Input: part model. Units: mm. Frame: model coordinates. A direction names the side the tool comes from. Give positions to 0.01 mm unless a question says otherwise; leave off trailing zeros. Order: outer loops, then holes, each group sorted by start corner. A loop starts at its lowest first (then second) coordinate and runs counter-clockwise, first axis right, second up. Notation, with made-up numbers: (82, 76) - (136, 76) arc R9 cw to (136, 86) - close; hole circle Ø10 at (7, 41.25). An arc over 180 degrees is marked (long way). Use a Markdown table: item, result.
from build123d import *

# Parameters (mm, degrees)
SKETCH013_W             = 28.2
SKETCH013_H             = 23.6
PAD004_DEPTH            = 2
SKETCH014_W             = 1.9812
SKETCH014_H             = 1.27
POCKET005_DEPTH         = 2
SKETCH015_R             = 4
SKETCH015_R_2           = 2.5
PAD005_DEPTH            = 8.6
SKETCH016_R             = 1.7
POCKET006_DEPTH         = 2
BODY002_PLACEMENT_ANGLE = 180


with BuildPart() as part:
    # Sketch013 → Pad004 (new body)
    with BuildSketch(Plane.XY):
        with Locations((0, -33.4375)):
            Rectangle(SKETCH013_W, SKETCH013_H)
    extrude(amount=PAD004_DEPTH)

    # Sketch014 (on Face6 of Pad004) → Pocket005 (cut)
    with BuildSketch(Plane.XY.offset(2)):
        with Locations((-6.1781, -26.6025)):
            Rectangle(SKETCH014_W, SKETCH014_H)
        with Locations((6.1781, -26.6025)):
            Rectangle(SKETCH014_W, SKETCH014_H)
    extrude(amount=-POCKET005_DEPTH, mode=Mode.SUBTRACT)

    # Sketch015 (on Face5 of Pocket005) → Pad005 (join)
    with BuildSketch(Plane.XY.offset(2)):
        with Locations((-6.1781, -26.6025)):
            Circle(SKETCH015_R)
        with Locations((-6.1781, -26.6025)):
            Circle(SKETCH015_R_2, mode=Mode.SUBTRACT)
        with Locations((6.1781, -26.6025)):
            Circle(SKETCH015_R)
        with Locations((6.1781, -26.6025)):
            Circle(SKETCH015_R_2, mode=Mode.SUBTRACT)
    extrude(amount=PAD005_DEPTH)

    # Sketch016 (on Face5 of Pad005) → Pocket006 (cut)
    with BuildSketch(Plane.XY.offset(2)):
        with Locations((-11, -42.2375)):
            Circle(SKETCH016_R)
        with Locations((11, -42.2375)):
            Circle(SKETCH016_R)
        with Locations((-11, -33.2375)):
            Circle(SKETCH016_R)
        with Locations((11, -33.2375)):
            Circle(SKETCH016_R)
    extrude(amount=-POCKET006_DEPTH, mode=Mode.SUBTRACT)


with BuildPart() as part_1:
    # Body002 placement: moved
    add(part.part.rotate(Axis((0, 0, 0), (0, 1, 0)), BODY002_PLACEMENT_ANGLE))


solid = part_1.part
1. Section query C-C (x = -3). Return loops of the section in (y, z).
Response:
| item | result |
|---|---|
| outline | (-45.24, -2) - (-29.03, -2) - (-29.03, -10.6) - (-24.17, -10.6) - (-24.17, -2) - (-21.64, -2) - (-21.64, 0) - (-45.24, 0) - close |
2. Section query B-B (z = -6.5). Return loops of the section in (x, y).
Response:
| item | result |
|---|---|
| outline | circle Ø8 at (-6.18, -26.6); circle Ø8 at (6.18, -26.6); hole circle Ø5 at (-6.18, -26.6); hole circle Ø5 at (6.18, -26.6) |
3. Section query A-A (x = 11). Return loops of the section in (y, z).
Response:
| item | result |
|---|---|
| outline | (-45.24, -2) - (-43.94, -2) - (-43.94, 0) - (-45.24, 0) - close; (-40.54, -2) - (-34.94, -2) - (-34.94, 0) - (-40.54, 0) - close; (-31.54, -2) - (-21.64, -2) - (-21.64, 0) - (-31.54, 0) - close |
4. Mould query, pull axis Y, two halves, no side actions, for faces 4 (the face through (-5.636, -29.043, -6.24)), 5 (the face through (-5.657, -22.637, -6.24)), 6 (the face through (-5.188, -27, -1)), 7 (the face through (-9, -27, -10.6)). Classes: pulls with the +Y half, pulls with the -Y half, needs draft (parallel to the pull), parting line crosses it, or undercut.
Response:
| item | result |
|---|---|
| face 4 | undercut |
| face 5 | parting line crosses it |
| face 6 | undercut |
| face 7 | needs draft |
5. Material intervals for line 1 along Y through (x, z) = (-11, -1.25); line 2 along Y through (x, z) = (-5.5, -1.5); line 3 along X through (y, z) = (-27.5, -7), sorted ascending.
Response:
| item | result |
|---|---|
| line 1 | y = -45.24 to -43.94, -40.54 to -34.94, -31.54 to -21.64 |
| line 2 | y = -45.24 to -27.24, -25.97 to -21.64 |
| line 3 | x = -10.08 to -8.51, -3.84 to -2.28, 2.28 to 3.84, 8.51 to 10.08 |
6. Pin query (flat end, axial travel): pin 1 (7 mm diameter, centred on x = 6, y = -32.5, fed in from -Z); pin 2 (1.5 mm diameter, centred on x = -7, y = -27, fed in from -Z). Return the tip coordinate at first contact, or that it passes through.
Response:
| item | result |
|---|---|
| pin 1 | stops at z = -10.6 |
| pin 2 | stops at z = -2 |
7. Section query D-D (z = -1.25). Return loops of the section in (x, y), then the cut area to 3 significant figures.
Response:
| item | result |
|---|---|
| outline | (-14.1, -45.24) - (14.1, -45.24) - (14.1, -21.64) - (-14.1, -21.64) - close; hole circle Ø3.4 at (-11, -42.24); hole circle Ø3.4 at (-11, -33.24); hole (-7.17, -27.24) - (-5.19, -27.24) - (-5.19, -25.97) - (-7.17, -25.97) - close; hole (5.19, -27.24) - (7.17, -27.24) - (7.17, -25.97) - (5.19, -25.97) - close; hole circle Ø3.4 at (11, -42.24); hole circle Ø3.4 at (11, -33.24) |
| area | 624 mm^2 |
8. Set-up query: faces 1 (the face through (5.188, -27, -1)), 2 (the face through (-6, -28, -2)), 3 (the face through (0, -21.638, -1)). Return all of +Z, -Z, +X, -X, +Y, -Y with unobstructed straight access to the full face (end or side cutting, diameter ignored); none if empty.
Response:
| item | result |
|---|---|
| face 1 | +Z, -Z |
| face 2 | -Z |
| face 3 | +Z, -Z, +X, -X, +Y |
